CAD build for the part. Positions are in the model's coordinates, mm. A direction names the side the tool comes from. Give positions to 0.01 mm unless a question says otherwise; leave off trailing zeros. Order: outer loops, then holes, each group sorted by start corner. A loop starts at its lowest first (then second) coordinate and runs counter-clockwise, first axis right, second up. Notation, with made-up numbers: (41, 29.25) -> (63, 29.25) arc R26 cw to (63, 57.25) -> close; hole circle Ø4 at (-32, -7). An arc over 180 degrees is marked (long way). Answer as CSV lines item,"result".
```python
from build123d import *

# Parameters (mm, degrees)
SKETCH_1_W           = 35
SKETCH_1_H           = 17
EXTRUDE_1_DEPTH      = 4
SKETCH_2_W           = 24
SKETCH_2_H           = 13
CUT_EXTRUDE_1_DEPTH  = 6
EXTRUDE_2_DEPTH      = 5
SKETCH_5_W           = 4
SKETCH_5_H           = 4
SKETCH_5_R           = 1.125
EXTRUDE_3_DEPTH      = 15
SKETCH_6_R           = 1.125
CUT_EXTRUDE_2_DEPTH  = 15
EXTRUDE_5_DEPTH      = 2
SKETCH_8_W           = 36
SKETCH_8_H           = 19
EXTRUDE_6_DEPTH      = 8.3
EXTRUDE_6_DEPTH_BACK = 10.7
SKETCH_9_W           = 24
SKETCH_9_H           = 13
CUT_EXTRUDE_3_DEPTH  = 22
SKETCH_11_R          = 1.125
CUT_EXTRUDE_4_DEPTH  = 15
CUT_EXTRUDE_5_DEPTH  = 15
SKETCH_13_W          = 3.77735738
SKETCH_13_H          = 19
CUT_EXTRUDE_6_DEPTH  = 8.5
SKETCH_14_W          = 10
SKETCH_14_H          = 5
CUT_EXTRUDE_7_DEPTH  = 10


with BuildPart() as part:
    # 草圖1 → 填料-伸長1 (new body)
    with BuildSketch(Plane.XY):
        with Locations((-3.721052632, 2.8)):
            Rectangle(SKETCH_1_W, SKETCH_1_H)
    extrude(amount=EXTRUDE_1_DEPTH)

    # 草圖2 → 除料-伸長1 (cut)
    with BuildSketch(Plane.XY):
        with Locations((-3.221052632, 2.8)):
            Rectangle(SKETCH_2_W, SKETCH_2_H)
    extrude(amount=CUT_EXTRUDE_1_DEPTH, mode=Mode.SUBTRACT)

    # 草圖3 → 填料-伸長2 (add)
    with BuildSketch(Plane(origin=(13.778947368, 0, 0), x_dir=(0, 0, -1), z_dir=(1, 0, 0))):
        Polygon((-4, 7.802538439), (-4, 11.3), (-19, 11.3), (-19, -5.694923122), (-4, -5.694923122), (-4, -2.197461561), (-9, -2.197461561), (-9, 7.802538439), align=None)
    extrude(amount=-EXTRUDE_2_DEPTH)

    # 草圖5 → 填料-伸長3 (add)
    with BuildSketch(Plane.XY.offset(4)):
        with Locations((-17.221052632, 2.8)):
            Rectangle(SKETCH_5_W, SKETCH_5_H)
        with Locations((-17.221052632, 2.8)):
            Circle(SKETCH_5_R, mode=Mode.SUBTRACT)
    extrude(amount=EXTRUDE_3_DEPTH)

    # 草圖6 → 除料-伸長2 (cut)
    with BuildSketch(Plane.XY.offset(19)):
        with Locations((11.278947368, 2.802538439)):
            Circle(SKETCH_6_R)
    extrude(amount=-CUT_EXTRUDE_2_DEPTH, mode=Mode.SUBTRACT)

    # 草圖7 → 填料-伸長5 (add)
    with BuildSketch(Plane.ZY.offset(21.221052632)):
        Polygon((4, 4.8), (4, 0.796544916), (19, 0.8), (19, 4.8), align=None)
    extrude(amount=-EXTRUDE_5_DEPTH)

    # 草圖8 → 填料-伸長6 (add, two sides)
    with BuildSketch(Plane(origin=(0, 3, 0), x_dir=(1, 0, 0), z_dir=(0, 1, 0))) as extrude_6_sk:
        with Locations((-39.221052632, -9.5)):
            Rectangle(SKETCH_8_W, SKETCH_8_H)
    extrude(amount=EXTRUDE_6_DEPTH)
    extrude(extrude_6_sk.sketch, amount=-EXTRUDE_6_DEPTH_BACK)

    # 草圖9 → 除料-伸長3 (cut)
    with BuildSketch(Plane(origin=(0, 11.3, 0), x_dir=(1, 0, 0), z_dir=(0, 1, 0))):
        with Locations((-40.998410012, -9.5)):
            Rectangle(SKETCH_9_W, SKETCH_9_H)
    extrude(amount=-CUT_EXTRUDE_3_DEPTH, mode=Mode.SUBTRACT)

    # 草圖11 → 除料-伸長4 (cut)
    with BuildSketch(Plane(origin=(0, -7.7, 0), x_dir=(-1, 0, 0), z_dir=(0, -1, 0))):
        with Locations((26.998410012, -9.5)):
            Circle(SKETCH_11_R)
        with Locations((54.999503046, -9.5)):
            Circle(SKETCH_11_R)
    extrude(amount=-CUT_EXTRUDE_4_DEPTH, mode=Mode.SUBTRACT)

    # 草圖12 → 除料-伸長5 (cut)
    with BuildSketch(Plane(origin=(0, -7.7, 0), x_dir=(-1, 0, 0), z_dir=(0, -1, 0))):
        Polygon((28.998410012, -7.5), (24.998410012, -7.5), (24.998410012, 0), (52.998410012, 0), (52.998410012, -3), (28.998410012, -3), align=None)
        Polygon((24.998410012, -11.5), (24.998410012, -19), (52.998410012, -19), (52.998410012, -16), (28.998410012, -16), (28.998410012, -11.5), align=None)
    extrude(amount=-CUT_EXTRUDE_5_DEPTH, mode=Mode.SUBTRACT)

    # 草圖13 → 除料-伸長6 (cut)
    with BuildSketch(Plane.XZ.offset(7.7)):
        with Locations((-23.109731322, 9.5)):
            Rectangle(SKETCH_13_W, SKETCH_13_H)
    extrude(amount=-CUT_EXTRUDE_6_DEPTH, mode=Mode.SUBTRACT)

    # 草圖14 → 除料-伸長7 (cut)
    with BuildSketch(Plane.ZY.offset(57.221052632)):
        with Locations((9.5, 4.8)):
            Rectangle(SKETCH_14_W, SKETCH_14_H)
    extrude(amount=-CUT_EXTRUDE_7_DEPTH, mode=Mode.SUBTRACT)


solid = part.part
```
1) Band-saw the part on A-A, the plane x = 3.5. Write the cut outline in (y, z).
Data:
outline,"(-5.7, 0) -> (-3.7, 0) -> (-3.7, 4) -> (-5.7, 4) -> close; (9.3, 0) -> (11.3, 0) -> (11.3, 4) -> (9.3, 4) -> close"
2) Pin check, flat tips, straight feed: P1, Ø3.5, axis at x = -55, y = 4.5, coming from the -Z side; P2, Ø3, axis at x = -16.5, z = 8.5, coming from the -Y side; P3, Ø4.5, axis at x = -28, y = -2, coming from the -Z side; P4, Ø0.7, axis at x = -26.5, z = 9.5, coming from the -Y side. Stop position of each tip, or through.
Data:
P1,"stops at z = 0"
P2,"stops at y = 0.8"
P3,"stops at z = 7.5"
P4,"stops at y = 7.3"
3) Wall check: line 1 along X through (y, z) = (-2.25, 9.5); line 2 along X through (y, z) = (3.5, 3); line 3 along X through (y, z) = (5.25, 17.5). Give the ranges that are in metal, low to high. Write a range as [from, to].
Data:
line 1,"x = [-57.22, -56.12], [-53.87, -53], [-29, -28.12], [-25.87, -25], [8.78, 13.78]"
line 2,"x = [-57.22, -53], [-25, -15.22], [8.78, 13.78]"
line 3,"x = [-57.22, -53], [-25, -21.22], [8.78, 13.78]"
4) Band-saw the part on B-B, the plane z = 17.75. Give the number of separate pieces and of enclosed holes in the cut face, then the cut area to 3 significant figures.
Data:
separate pieces,"2"
enclosed holes,"2"
area,"333 mm2"
5) Which spindle directions (+Z, -Z, +X, -X, +Y, -Y) get a long thin tool onto all of the face, cutting with end or side? Do faces 1 (the flat face through (-21.221, -2, 2)), 2 (the flat face through (11, -2.197, 6)), 3 (the flat face through (-55, 2.3, 8)), 4 (the flat face through (-41, 9, 3)). Say none if no direction does.
Data:
face 1,"+Z, -Z, -Y"
face 2,"+X"
face 3,"-X"
face 4,"+Y, -Y"
6) Pull direction Z, two halves, no side cores. Call faces 5 (the flat face through (-41, 7.5, 19)), 6 (the flat face through (11, 7.803, 7)), 7 (the flat face through (-27, 0, 7.5)): pulls with the +Z half, pulls with the -Z half, needs draft (parallel to the pull), parting line crosses it, or undercut.
Data:
face 5,"pulls with the +Z half"
face 6,"undercut"
face 7,"pulls with the -Z half"
7) Band-saw the part on C-C, the plane x = -49. Write the cut outline in (y, z), then the cut area to 3 significant figures.
Data:
outline,"(7.3, 0) -> (11.3, 0) -> (11.3, 3) -> (7.3, 3) -> close; (7.3, 16) -> (11.3, 16) -> (11.3, 19) -> (7.3, 19) -> close"
area,"24.0 mm2"
